The listing builds one solid part. Answer for the finished solid, in the listing's coordinates (mm). Coordinates: 2 decimals unless noted, no trailing zeros. Write each question's results on one line, items separated by ' | '. Start each with the question number.
(1) Given pin 1 Ø10 at (x, y) = (274.5, -253) entering from -Z; pin 2 Ø8 at (y, z) = (-63.5, -17) entering from +X; pin 3 Ø10 at (x, z) = (-708.5, 25) entering from +Y, each flat-ended and moving along its own axis, determine where each tip first touches the part or whether it passes through.
(2) Consider line 1 (Y direction, x = -900, z = -14); line 2 (Y direction, x = -632, z = -1.5); line 3 (X direction, y = -479, z = 0). Determine where each line is inside the solid, lowest interval first. Write a range as from..to.
(3) Find section A-A on x = 401.5. State how many separate pieces and enclosed holes the cut face has, then the cut area to 3 significant figures.
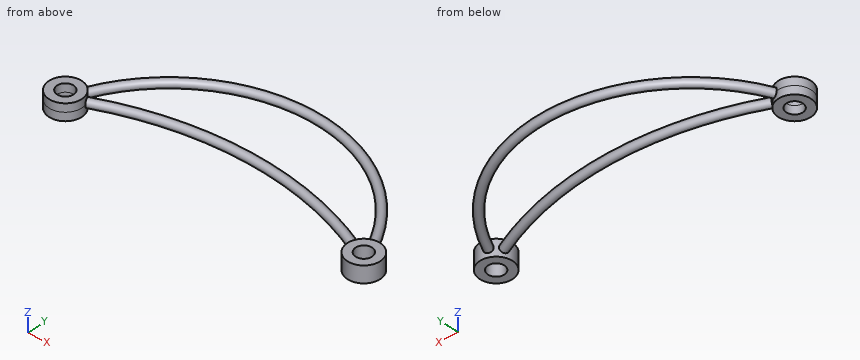
from build123d import *

# Parameters (mm, degrees)
F2_R     = 25.4
F2_R_2   = 21.742
F3_R     = 25.4
F3_R_2   = 21.742
F6_R     = 100
F6_R_2   = 50
F7_DEPTH = 50


with BuildPart() as f4:
    # F4: sweep along a path in F1
    with BuildLine(Plane.XY) as f4_path:
        ThreePointArc((810.7144863791, -440.4517624252), (0, -258.8062140954), (-810.7144863791, -440.4517624252))
    # F2 (on Right) → F4 (sweep)
    with BuildSketch(Plane.YZ):
        with Locations((-258.8062140954, 0)):
            Circle(F2_R)
        with Locations((-258.8062140954, 0)):
            Circle(F2_R_2, mode=Mode.SUBTRACT)
    sweep(path=f4_path.line)



with BuildPart() as f5:
    # F5: sweep along a path in F1
    with BuildLine(Plane.XY) as f5_path:
        ThreePointArc((863.0516210993, -392.5624434058), (0, 160.4350098154), (-863.0516210993, -392.5624434058))
    # F3 (on Right) → F5 (sweep)
    with BuildSketch(Plane.YZ):
        with Locations((160.4350098154, 0)):
            Circle(F3_R)
        with Locations((160.4350098154, 0)):
            Circle(F3_R_2, mode=Mode.SUBTRACT)
    sweep(path=f5_path.line)


with BuildPart() as f4_1:
    add(f4.part)

    add(f5.part)  # F7 merges F5
    # F6 (on Top) → F7 (join, symmetric)
    with BuildSketch(Plane.XY):
        with Locations((-900, -485.4861610273)):
            Circle(F6_R)
        with Locations((-900, -485.4861610273)):
            Circle(F6_R_2, mode=Mode.SUBTRACT)
        with Locations((900, -485.4861610273)):
            Circle(F6_R)
        with Locations((900, -485.4861610273)):
            Circle(F6_R_2, mode=Mode.SUBTRACT)
    extrude(amount=F7_DEPTH, both=True)


solid = f4_1.part
Values:
1) pin 1: stops at z = -15.03 | pin 2: stops at x = 648.01 | pin 3: stops at y = -132.05
2) line 1: y = -585.49..-535.49, -435.49..-385.49 | line 2: y = -393.91..-390.01, -344.01..-340.13, -114.64..-109.62, -51.5..-46.68 | line 3: x = -999.79..-949.58, -850.42..-800.21, 800.21..850.42, 949.58..999.79
3) separate pieces: 2 | enclosed holes: 2 | area: 1,150 mm²
